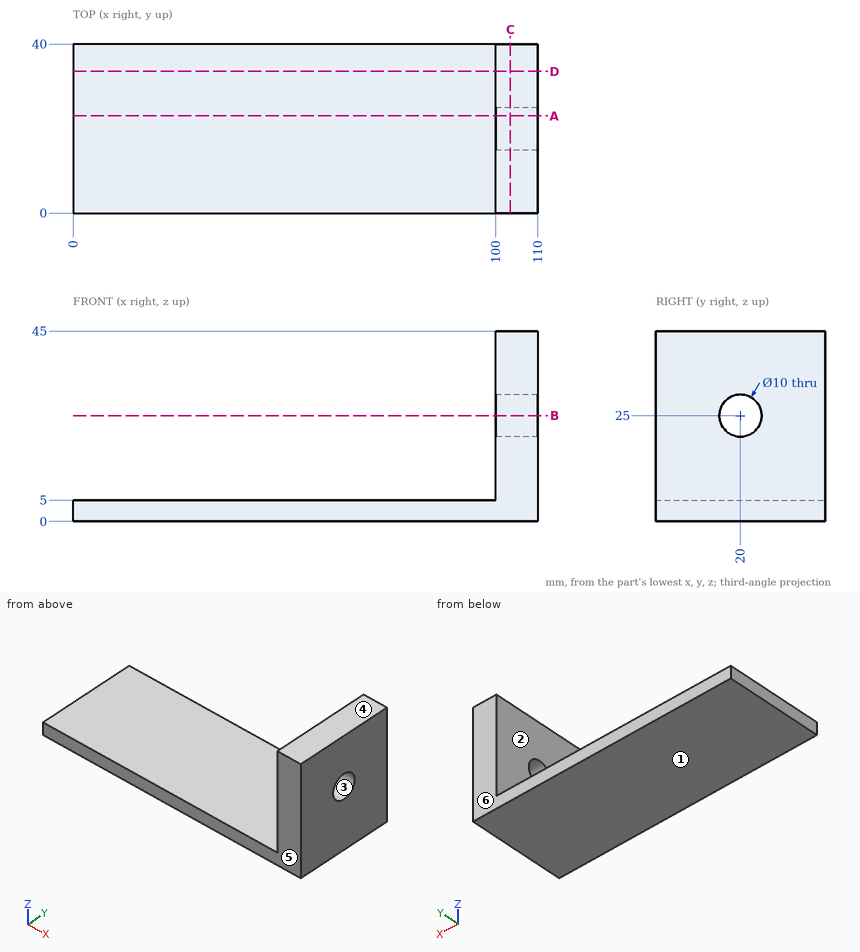
Here's the drawing with two shaded views (mm, measured from the low corner). I have some questions. A direction names the side the tool comes from. Round coordinates to 2 decimals unless told otherwise and drop trailing zeros. Write each loop counter-clockwise with the first axis right and the second up, starting at its lowest first coordinate (ties: lowest second). Pieces come first, ordered by that corner, then holes. Notation, with made-up numbers: M 78,61 L 97,61 A30 cw 97,89 Z; hole C -30,28 d1. An arc over 180 degrees is marked long. Write each question's results on one line, items separated by ' | '. Start each with the question number.
1. Imagine slicing it at B-B on z = 25. List the corners of the cut face in (x, y) for me.
2. Imagine slicing it at C-C on x = 103.5. List the corners of the cut face in (y, z) for me, and give its area (3 significant figures).
3. On a 3-axis mill with a long thin cutter (end or side, diameter ignored), from which of +Z, -Z, +X, -X, +Y, -Y can I reach the whole of each face in a straight line? I mean the marked faces 1 and 2. Say none if no direction works.
4. I need wall thicknesses on L1, parallel to Z at x = 107.75, y = 20; L2, parallel to Y at x = 106.75, z = 25; L3, parallel to X at y = 2.5, z = 9.5. Which ranges of each line are inside material? Lowest first, please. Write a range as from..to.
5. Imagine slicing it at A-A on y = 23. List the corners of the cut face in (x, z) for me.
6. Imagine slicing it at D-D on y = 33.5. List the corners of the cut face in (x, z) for me, and give its area (3 significant figures).
7. Thinking about a two-plate mould opening in Y: for the marked faces 3, 4, 5 and 6, which applies, +Y half, -Y half, draft (parallel to the pull), parting line (faces both ways), or undercut?
8. I'm going to push a flat-ended pin straight in: pin 1 Ø6 at (y, z) = (18, 19) entering from -X. Where does the tip first touch, or does it pass through?
Result sheet:
1) outline: M 100,0 L 110,0 L 110,15 L 100,15 Z; M 100,25 L 110,25 L 110,40 L 100,40 Z
2) outline: M 0,0 L 40,0 L 40,45 L 0,45 Z; hole C 20,25 d10 | area: 1,720 mm^2
3) face 1: -Z, +X, -X, +Y, -Y | face 2: +Z, -X, +Y, -Y
4) L1: z = 0..20, 30..45 | L2: y = 0..15, 25..40 | L3: x = 100..110
5) outline: M 0,0 L 110,0 L 110,21 L 100,21 L 100,5 L 0,5 Z; M 100,29 L 110,29 L 110,45 L 100,45 Z
6) outline: M 0,0 L 110,0 L 110,45 L 100,45 L 100,5 L 0,5 Z | area: 950 mm^2
7) face 3: undercut | face 4: draft | face 5: -Y half | face 6: +Y half
8) pin 1: stops at x = 100
